Read the model definition and answer for the solid it produces. Units are mm, in the model's axes. Face numbers are marked on the shaded views. Give positions to 0.01 mm unless a question says otherwise; leave off trailing zeros. Write each loop counter-clockwise with the first axis right and the second up, starting at its lowest first coordinate (ties: lowest second). Pieces come first, ordered by that corner, then holes. Notation, with made-up numbers: (2.25, 73) - (58.25, 73) arc R7 ccw to (58.25, 86) - close; hole circle Ø11 at (35, 50.25). An arc over 180 degrees is marked (long way). Answer as CSV lines item,"result".
```python
from build123d import *

# Parameters (mm, degrees)
F0_W     = 228.6
F0_H     = 127
F0_R     = 19.492396
F1_DEPTH = 76.2
F2_R     = 5.08
F3_R     = 5.08
F4_DEPTH = 25.4


with BuildPart() as f1:
    # F0 (on Top) → F1 (new body)
    with BuildSketch(Plane.XY):
        Rectangle(F0_W, F0_H)
        with Locations((77.086605, -29.871058)):
            Circle(F0_R, mode=Mode.SUBTRACT)
    extrude(amount=F1_DEPTH)

    # F2
    f2_edges = [f1.edges().sort_by_distance(p)[0] for p in [
        (-114.3, 63.5, 38.1),
        (-114.3, -63.5, 38.1),
        (-114.3, 0, 0),
        (-114.3, 0, 76.2),
    ]]
    fillet(f2_edges, radius=F2_R)

    # F3
    f3_edges = [f1.edges().sort_by_distance(p)[0] for p in [
        (114.3, -63.5, 38.1),
        (114.3, 63.5, 38.1),
        (114.3, 0, 0),
        (114.3, 0, 76.2),
    ]]
    fillet(f3_edges, radius=F3_R)

    # F0 (on Top) → F4 (cut)
    with BuildSketch(Plane.XY):
        with Locations((77.086605, -29.871058)):
            Circle(F0_R)
    extrude(amount=F4_DEPTH, mode=Mode.SUBTRACT)


solid = f1.part
```
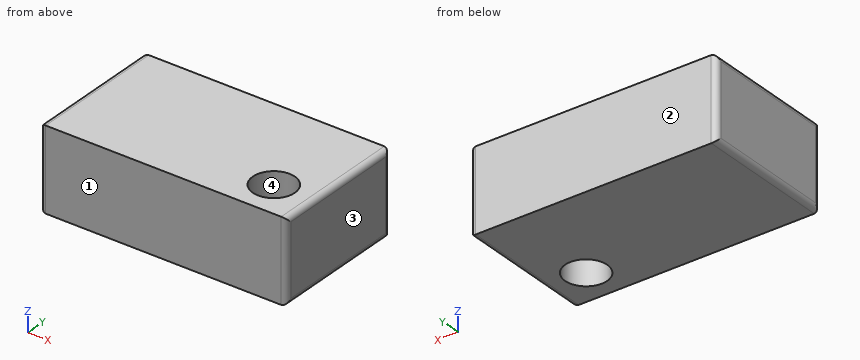
(1) A cutting plane is placed at C-C (z = 55). Write down the section's boundary in (x, y).
Worked out:
outline,"(-114.3, -58.42) arc R5.08 ccw to (-109.22, -63.5) - (109.22, -63.5) arc R5.08 ccw to (114.3, -58.42) - (114.3, 58.42) arc R5.08 ccw to (109.22, 63.5) - (-109.22, 63.5) arc R5.08 ccw to (-114.3, 58.42) - close; hole circle Ø38.98 at (77.09, -29.87)"
(2) A cutting plane is placed at B-B (x = 64). Write down the section's boundary in (y, z).
Worked out:
outline,"(-63.5, 0) - (-44.32, 0) - (-44.32, 76.2) - (-63.5, 76.2) - close; (-15.42, 0) - (63.5, 0) - (63.5, 76.2) - (-15.42, 76.2) - close"
(3) A cutting plane is placed at A-A (y = -37). Write down the section's boundary in (x, z), and give its area (3 significant figures).
Worked out:
outline,"(-114.3, 5.08) arc R5.08 ccw to (-109.22, 0) - (58.94, 0) - (58.94, 76.2) - (-109.22, 76.2) arc R5.08 ccw to (-114.3, 71.12) - close; (95.23, 0) - (109.22, 0) arc R5.08 ccw to (114.3, 5.08) - (114.3, 71.12) arc R5.08 ccw to (109.22, 76.2) - (95.23, 76.2) - close"
area,"14,600 mm^2"
(4) Find the intervals of material crossed by L1, parallel to X at y = -21.5, z = 5.5; L2, parallel to X at y = -19.5, z = 12; L3, parallel to Y at x = 59.5, z = 13, in increasing order.
Worked out:
L1,"x = -114.3 to 59.48, 94.69 to 114.3"
L2,"x = -114.3 to 60.58, 93.59 to 114.3"
L3,"y = -63.5 to -38.28, -21.46 to 63.5"
(5) The mould has two halves that part along Y. Classify the marked faces 1, 2, 3 and 4: +Y half, -Y half, draft (parallel to the pull), parting line (faces both ways), or undercut.
Worked out:
face 1,"-Y half"
face 2,"+Y half"
face 3,"draft"
face 4,"undercut"
